Input: part model. Units: mm. Frame: model coordinates. A direction names the side the tool comes from. Round coordinates to 2 decimals unless told otherwise and drop trailing zeros. Loops run counter-clockwise (first coordinate to the right, second up) from the corner with the lowest first, then second, coordinate; pieces in that order, holes last. Notation, with made-up numbers: (62, 60.25) -> (71, 60.25) arc R23 ccw to (71, 68.25) -> close; hole circle Ø11 at (-9, 44.25). An arc over 180 degrees is marked (long way). Answer as a JSON object with one key per item and string values.
```python
from build123d import *

# Parameters (mm, degrees)
SKETCH1_R               = 25
BOSS_EXTRUDE1_DEPTH     = 5
BOSS_EXTRUDE2_DEPTH     = 34.79
SKETCH3_W               = 21.3
SKETCH3_H               = 5
BOSS_EXTRUDE3_DEPTH     = 25
SKETCH4_W               = 3
SKETCH4_H               = 29.79
BOSS_EXTRUDE5_DEPTH     = 5
CUT_EXTRUDE1_DEPTH      = 38
CUT_EXTRUDE1_DEPTH_BACK = 50.601855812
SKETCH5_R               = 1
FILLET1_R               = 1
FILLET2_R               = 1
FILLET3_R               = 1
CUT_EXTRUDE2_REACH      = 55.228
CUT_EXTRUDE2_END_RADIUS = 1
SKETCH6_R               = 0.5


with BuildPart() as part:
    # Sketch1 → Boss-Extrude1 (new body)
    with BuildSketch(Plane.XY):
        Circle(SKETCH1_R)
    extrude(amount=-BOSS_EXTRUDE1_DEPTH)

    # Sketch2 → Boss-Extrude2 (add)
    with BuildSketch(Plane.XY):
        with BuildLine():
            Line((-10.65, -10.65), (10.65, -10.65))
            ThreePointArc((10.65, -10.65), (10.553147336, -12.083032205), (10.264350929, -13.49))
            Line((10.264350929, -13.49), (-10.264350929, -13.49))
            ThreePointArc((-10.264350929, -13.49), (-10.553147336, -12.083032205), (-10.65, -10.65))
        make_face()
    extrude(amount=BOSS_EXTRUDE2_DEPTH)

    # Sketch3 → Boss-Extrude3 (add)
    with BuildSketch(Plane(origin=(0, -10.65, 0), x_dir=(1, 0, 0), z_dir=(0, 1, 0))):
        with Locations((0, -32.29)):
            Rectangle(SKETCH3_W, SKETCH3_H)
    extrude(amount=BOSS_EXTRUDE3_DEPTH)

    # Sketch4 → Boss-Extrude5 (add)
    with BuildSketch(Plane(origin=(0, -10.65, 0), x_dir=(1, 0, 0), z_dir=(0, 1, 0))):
        with Locations((9, -14.895)):
            Rectangle(SKETCH4_W, SKETCH4_H)
        with Locations((-9, -14.895)):
            Rectangle(SKETCH4_W, SKETCH4_H)
    extrude(amount=BOSS_EXTRUDE5_DEPTH)

    # Sketch5 → Cut-Extrude1 (cut, two sides: drawn at the far end of the back side and taken through both)
    with BuildSketch(Plane(origin=(0, 0, 0), x_dir=(1, 0, 0), z_dir=(0, 1, 0)).offset(-CUT_EXTRUDE1_DEPTH_BACK)):
        with Locations(Location((0, 2.5, 0), (0, 0, 90))):
            Circle(SKETCH5_R)
    extrude(amount=CUT_EXTRUDE1_DEPTH + CUT_EXTRUDE1_DEPTH_BACK, mode=Mode.SUBTRACT)

    # Fillet1
    fillet1_edges = [part.edges().sort_by_distance(p)[0] for p in [
        (10.65, 14.35, 32.29),
        (-10.65, 14.35, 32.29),
    ]]
    fillet(fillet1_edges, radius=FILLET1_R)

    # Fillet2
    fillet2_edges = [part.edges().sort_by_distance(p)[0] for p in [
        (7.5, -10.65, 14.895),
        (-7.5, -10.65, 14.895),
    ]]
    fillet(fillet2_edges, radius=FILLET2_R)

    # Fillet3
    # the kernel refuses this fillet: 1 mm, written as the material it adds along each edge
    with BuildSketch(Plane(origin=(10.5, -10.65, 31.106956719), x_dir=(0, 1, 0), z_dir=(0, 0, -1))) as fillet3_piece_1:
        with BuildLine():
            CenterArc((0.526782688, 1), FILLET3_R, 238.211669382, 31.788330618)
            Line((0, 0.15), (-0.010535654, 0.133))
            ThreePointArc((-0.010535654, 0.133), (-0.02, 0.075), (-0.02, 0))
            Line((-0.02, 0), (0, -0.02))
            Line((0, -0.02), (0.526782688, -0.02))
            Line((0.526782688, -0.02), (0.526782688, 0))
        make_face()
    extrude(amount=32.423913438)
    with BuildSketch(Plane(origin=(-10.5, -10.65, 31.106956719), x_dir=(0, 1, 0), z_dir=(0, 0, -1))) as fillet3_piece_2:
        with BuildLine():
            CenterArc((0.526782688, -1), FILLET3_R, 90, 31.788330618)
            Line((0, -0.15), (-0.010535654, -0.133))
            ThreePointArc((-0.010535654, -0.133), (-0.02, -0.075), (-0.02, 0))
            Line((-0.02, 0), (0, 0.02))
            Line((0, 0.02), (0.526782688, 0.02))
            Line((0.526782688, 0.02), (0.526782688, 0))
        make_face()
    extrude(amount=32.423913438)

    # Cut-Extrude2: up to this cylinder (the profile starts outside it)
    cut_extrude2_end = Plane(origin=(0, 0, -2.5), z_dir=(0, -1, 0)) * Cylinder(CUT_EXTRUDE2_END_RADIUS, 135.456, mode=Mode.PRIVATE)
    # Sketch6 → Cut-Extrude2 (cut, up to the surface)
    with BuildSketch(Plane(origin=(0, 0, -5), x_dir=(-1, 0, 0), z_dir=(0, 0, -1)), mode=Mode.PRIVATE) as cut_extrude2_sk1:
        with Locations((0, 11)):
            Circle(SKETCH6_R)
    cut_extrude2_tool1 = extrude(cut_extrude2_sk1.sketch, amount=-CUT_EXTRUDE2_REACH, mode=Mode.PRIVATE) - cut_extrude2_end
    add(cut_extrude2_tool1.solids().sort_by_distance((0, 11, -5))[0], mode=Mode.SUBTRACT)
    # Sketch6 → Cut-Extrude2 (cut, up to the surface)
    with BuildSketch(Plane(origin=(0, 0, -5), x_dir=(-1, 0, 0), z_dir=(0, 0, -1)), mode=Mode.PRIVATE) as cut_extrude2_sk2:
        with Locations((0, -11)):
            Circle(SKETCH6_R)
    cut_extrude2_tool2 = extrude(cut_extrude2_sk2.sketch, amount=-CUT_EXTRUDE2_REACH, mode=Mode.PRIVATE) - cut_extrude2_end
    add(cut_extrude2_tool2.solids().sort_by_distance((0, -11, -5))[0], mode=Mode.SUBTRACT)


solid = part.part
```
1) Section C-C, the plane y = -20.5. Output: boundary loops of the cut face in (x, z).
Output:
{"outline": "(-14.31, -5) -> (14.31, -5) -> (14.31, 0) -> (-14.31, 0) -> close; hole circle Ø2 at (0, -2.5)"}
2) Ray query, probe 1 along Y at (x, z) = (0, -4.25); probe 2 along Z at (x, y) = (10, 8); probe 3 along Y at (x, z) = (-9, 27). Return the intervals inside material, ascending.
Output:
{"probe 1": "y = -25 to -11.5, -10.5 to 10.5, 11.5 to 25", "probe 2": "z = -5 to 0, 29.79 to 34.79", "probe 3": "y = -13.49 to -5.65"}
3) Section D-D, the plane z = -2.5. Output: boundary loops of the cut face in (x, y).
Output:
{"outline": "(-1, -24.98) -> (-1, 24.98) arc R25 ccw to start; (1, -24.98) arc R25 ccw to (1, 24.98) -> close"}
4) Section A-A, the plane y = 0. Output: boundary loops of the cut face in (x, z), plus the area to 3 significant figures.
Output:
{"outline": "(-25, -5) -> (25, -5) -> (25, 0) -> (-25, 0) -> close; (-10.65, 29.79) -> (10.65, 29.79) -> (10.65, 34.79) -> (-10.65, 34.79) -> close; hole circle Ø2 at (0, -2.5)", "area": "353 mm^2"}
5) Reachability of faces 1 (the face through (0, 14.35, 32)), 2 (the face through (10.5, -8, 15)), 3 (the face through (9, -5.65, 15)), 4 (the face through (-10.55, -12.1, 17.15)), 5 (the face through (0, 2, 29.79)) from +Z, -Z, +X, -X, +Y, -Y: full face, straight path, thin tool, end or side. Return the list, or none.
Output:
{"face 1": "+Z, +X, -X, +Y", "face 2": "+X, +Y", "face 3": "+X, -X, +Y", "face 4": "+Z, -X, -Y", "face 5": "+Y"}
6) Contact query for flat-ended pins moving along their axis: P1, Ø4, axis at y = -4, z = 33.5, coming from the +X side; P2, Ø6, axis at x = 3, z = 11, coming from the -Y side; P3, Ø3.5, axis at x = -9, z = 10.5, coming from the +Y side; P4, Ø5, axis at x = -13, y = -0.5, coming from the +Z side. Output: stop coordinate, or through.
Output:
{"P1": "stops at x = 10.65", "P2": "stops at y = -13.49", "P3": "stops at y = -5.65", "P4": "stops at z = 34.79"}
7) Section B-B, the plane z = 14. Output: boundary loops of the cut face in (x, y), plus the area to 3 significant figures.
Output:
{"outline": "(-10.65, -10.65) arc R10.65 ccw to (-10.26, -13.49) -> (10.26, -13.49) arc R10.65 ccw to (10.65, -10.65) arc R1 cw to (10.5, -10.12) -> (10.5, -5.65) -> (7.5, -5.65) -> (7.5, -9.65) arc R1 cw to (6.5, -10.65) -> (-6.5, -10.65) arc R1 cw to (-7.5, -9.65) -> (-7.5, -5.65) -> (-10.5, -5.65) -> (-10.5, -10.12) arc R1 cw to start", "area": "90.2 mm^2"}
8) Draft query along Z for faces 6 (the face through (0, 0, -5)), 7 (the face through (10.65, 1, 32)), 8 (the face through (0, 0, 34.79)), 9 (the face through (7.5, -8, 15)). Return one class per face: +Z half, -Z half, draft (parallel to the pull), parting line (faces both ways), or undercut.
Output:
{"face 6": "-Z half", "face 7": "draft", "face 8": "+Z half", "face 9": "undercut"}
